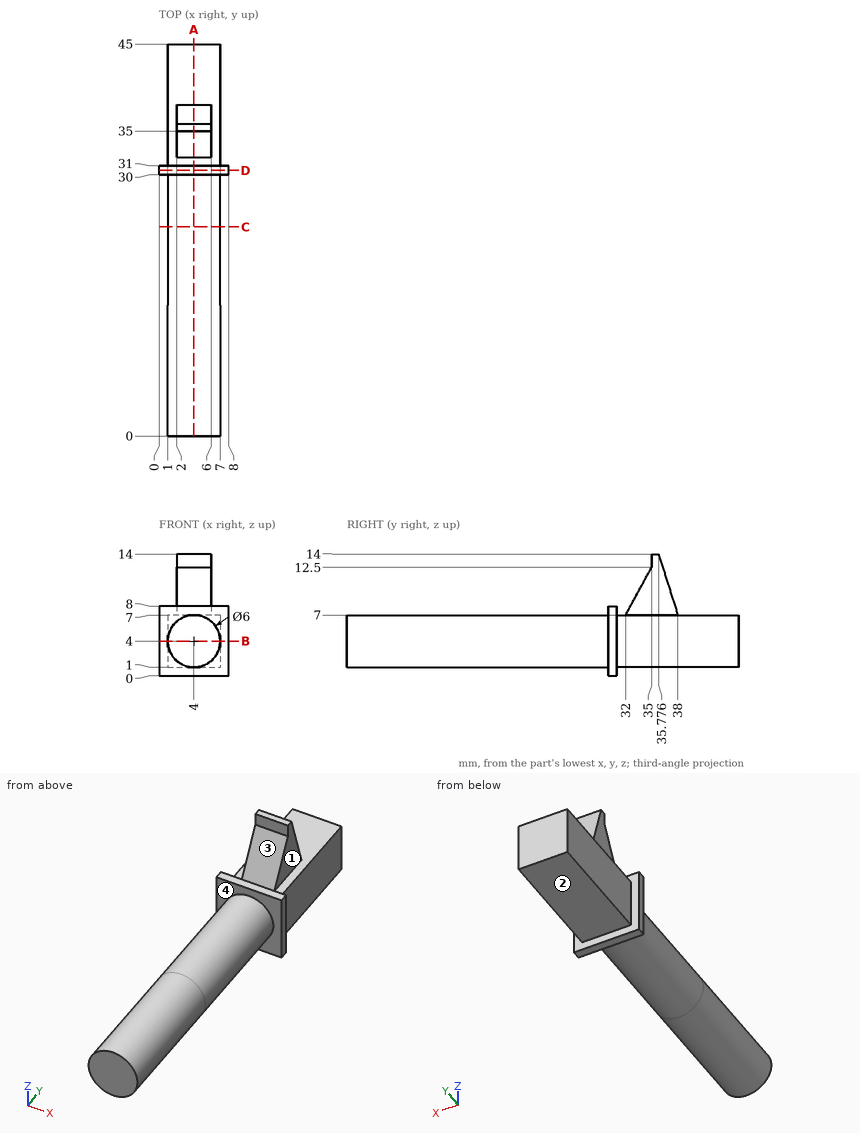
Design review of the part shown in the three views and the two pictorial views. Dimensions are in mm from the part's minimum x, y and z. A direction names the side the tool comes from. Give positions to 0.01 mm unless a question says otherwise; leave off trailing zeros. Write each loop counter-clockwise with the first axis right and the second up, starting at its lowest first coordinate (ties: lowest second). Pieces come first, ordered by that corner, then holes. Notation, with made-up numbers: (52.25, 76.5) - (103.25, 76.5) arc R16 ccw to (103.25, 84.5) - close; hole circle Ø9 at (-34, 22.25). An arc over 180 degrees is marked (long way). Return JSON: item names as keys, results as strings. Group by question number.
(1) We need section C-C, the plane y = 24. Give the boundary of the cut face in (x, z).
(2) To check wall thickness, follow probe 1 along X at (y, z) = (19, 4); probe 2 along Y at (x, z) = (6.5, 0.5); probe 3 along X at (y, z) = (36.5, 9.5). State the ranges of each line that lie inside material, in increasing order.
(3) Insertion check: pin 1 (1.8 mm diameter, centred on y = 35, z = 4, fed in from -X); pin 2 (1.8 mm diameter, centred on y = 39, z = 3.5, fed in from +X); pin 3 (2 mm diameter, centred on y = 7.5, z = 9, fed in from +X); pin 4 (0.8 mm diameter, centred on x = 3.5, y = 30.5, fed in from +Z). Each pin has a flat end and moves straight along its axis. Give the tip position at first contact, or say it passes through.
(4) We need section D-D, the plane y = 30.5. Give the boundary of the cut face in (x, z).
(5) We need section A-A, the plane x = 4. Give the boundary of the cut face in (y, z).
(6) Machinability: for the marked faces 1, 2, 3 and 4, which of the approach directions +Z, -Z, +X, -X, +Y, -Y give a long, thin tool a straight path to every point of the face, cutting with its end or side? Answer none if there is none.
(7) We need section B-B, the plane z = 4. Give the boundary of the cut face in (x, y).
Reported:
{
 "1": {"outline": "circle Ø6 at (4, 4)"},
 "2": {"probe 1": "x = 1 to 7", "probe 2": "y = 30 to 31", "probe 3": "x = 2 to 6"},
 "3": {"pin 1": "stops at x = 1", "pin 2": "stops at x = 7", "pin 3": "passes through", "pin 4": "stops at z = 8"},
 "4": {"outline": "(0, 0) - (8, 0) - (8, 8) - (0, 8) - close"},
 "5": {"outline": "(0, 1) - (30, 1) - (30, 0) - (31, 0) - (31, 1) - (45, 1) - (45, 7) - (38, 7) - (35.78, 14) - (35, 14) - (35, 12.5) - (32, 7) - (31, 7) - (31, 8) - (30, 8) - (30, 7) - (0, 7) - close"},
 "6": {"face 1": "+Z, +X, +Y", "face 2": "-Z, +X, -X, +Y", "face 3": "+Z, +X, -X", "face 4": "-Y"},
 "7": {"outline": "(0, 30) - (1, 30) - (1, 0) - (7, 0) - (7, 30) - (8, 30) - (8, 31) - (7, 31) - (7, 45) - (1, 45) - (1, 31) - (0, 31) - close"}
}
